from build123d import *

# Parameters (mm, degrees)
BOSS_EXTRUDE1_DEPTH = 30
SKETCH3_R           = 1.6
CUT_EXTRUDE1_DEPTH  = 10
SKETCH2_R           = 6
CUT_EXTRUDE2_DEPTH  = 10
CHAMFER1_SIZE       = 2


with BuildPart() as part:
    # Sketch1 → Boss-Extrude1 (new body)
    with BuildSketch(Plane.XY):
        Polygon((0, 0), (30, 0), (30, 1), (1, 1), (1, 28), (30, 28), (30, 29), (0, 29), (0, 28), (0, 1), align=None)
    extrude(amount=BOSS_EXTRUDE1_DEPTH)

    # Sketch3 → Cut-Extrude1 (cut)
    with BuildSketch(Plane(origin=(0, 29, 0), x_dir=(1, 0, 0), z_dir=(0, 1, 0))):
        with Locations(Location((19.603232535, -19.78053164, 0), (0, 0, 270))):
            Circle(SKETCH3_R)
        with Locations(Location((9.308321888, -16.163237793, 0), (0, 0, 270))):
            Circle(SKETCH3_R)
        with Locations(Location((17.588445577, -9.056230567, 0), (0, 0, 270))):
            Circle(SKETCH3_R)
    extrude(amount=-CUT_EXTRUDE1_DEPTH, mode=Mode.SUBTRACT)

    # Sketch2 → Cut-Extrude2 (cut)
    with BuildSketch(Plane(origin=(0, 1, 0), x_dir=(1, 0, 0), z_dir=(0, 1, 0))):
        with Locations(Location((15.5, -15, 0), (0, 0, 270))):
            Circle(SKETCH2_R)
    extrude(amount=-CUT_EXTRUDE2_DEPTH, mode=Mode.SUBTRACT)

    # Chamfer1
    chamfer1_edges = [part.edges().sort_by_distance(p)[0] for p in [
        (30, 28.5, 0),
        (30, 0.5, 30),
        (30, 0.5, 0),
        (30, 28.5, 30),
    ]]
    chamfer(chamfer1_edges, length=CHAMFER1_SIZE)


solid = part.part
Geometry check sheet. Reference: the model listing, model coordinates, mm. A direction names the side the tool comes from. Round coordinates to 2 decimals unless told otherwise and drop trailing zeros. Loops run counter-clockwise (first coordinate to the right, second up) from the corner with the lowest first, then second, coordinate; pieces in that order, holes last. Notation, with made-up numbers: (64, -28) -> (84, -28) arc R12 ccw to (84, -5) -> close; hole circle Ø1 at (43.25, 33.25). An arc over 180 degrees is marked (long way). Answer as a JSON object with one key per item and string values. Group by question number.
Item 1: Release check for a two-part mould opening along Y. For faces 1 (the face through (29, 0.5, 1)), 2 (the face through (15, 29, 15)), 3 (the face through (1, 14, 15)) record: pulls with the +Y half, pulls with the -Y half, needs draft (parallel to the pull), parting line crosses it, or undercut.
Item 2: Thickness scan on line 1 along Y through (x, z) = (11, 10); line 2 along X through (y, z) = (17.5, 20.5); line 3 along Y through (x, z) = (18, 17.5). Record the ranges inside material, lowest first.
Item 3: Cross-section at A-A, the plane x = 15.5. Record the cut outline in (y, z), plus the area to 3 significant figures.
Item 4: Cross-section at C-C, the plane z = 25.75. Record the cut outline in (x, y), plus the area to 3 significant figures.
Item 5: Cross-section at D-D, the plane z = 12. Record the cut outline in (x, y).
Item 6: Cross-section at B-B, the plane z = 15. Record the cut outline in (x, y).
Item 7: Set-up check for faces 4 (the face through (15, 28, 15)), 5 (the face through (30, 0.5, 14.8)), 6 (the face through (18.938, 28.507, 9.916)), 7 (the face through (17.302, 0.507, 20.723)): record each of +Z, -Z, +X, -X, +Y, -Y from which the full face is reachable in a straight line by a thin tool's end or side.
Item 8: Depth check by flat-ended pin: pin 1 Ø13.5 at (y, z) = (16, 10) entering from +X; pin 2 Ø2.5 at (x, z) = (9.31, 16.16) entering from +Y. Enter the tip coordinate at first touch or a pass-through.
Determined:
{
 "1": {"face 1": "needs draft", "face 2": "pulls with the +Y half", "face 3": "undercut"},
 "2": {"line 1": "y = 0 to 1, 28 to 29", "line 2": "x = 0 to 1", "line 3": "y = 28 to 29"},
 "3": {"outline": "(0, 0) -> (1, 0) -> (1, 9) -> (0, 9) -> close; (0, 21) -> (1, 21) -> (1, 30) -> (0, 30) -> close; (28, 0) -> (29, 0) -> (29, 30) -> (28, 30) -> close", "area": "48.0 mm²"},
 "4": {"outline": "(0, 0) -> (30, 0) -> (30, 1) -> (1, 1) -> (1, 28) -> (30, 28) -> (30, 29) -> (0, 29) -> close", "area": "87.0 mm²"},
 "5": {"outline": "(0, 0) -> (10.3, 0) -> (10.3, 1) -> (1, 1) -> (1, 28) -> (30, 28) -> (30, 29) -> (0, 29) -> close; (20.7, 0) -> (30, 0) -> (30, 1) -> (20.7, 1) -> close"},
 "6": {"outline": "(0, 0) -> (9.5, 0) -> (9.5, 1) -> (1, 1) -> (1, 28) -> (8.21, 28) -> (8.21, 29) -> (0, 29) -> close; (10.41, 28) -> (30, 28) -> (30, 29) -> (10.41, 29) -> close; (21.5, 0) -> (30, 0) -> (30, 1) -> (21.5, 1) -> close"},
 "7": {"face 4": "+Z, -Z, +X", "face 5": "+Z, -Z, +X, +Y, -Y", "face 6": "+Y", "face 7": "-Y"},
 "8": {"pin 1": "stops at x = 1", "pin 2": "stops at y = 1"}
}
